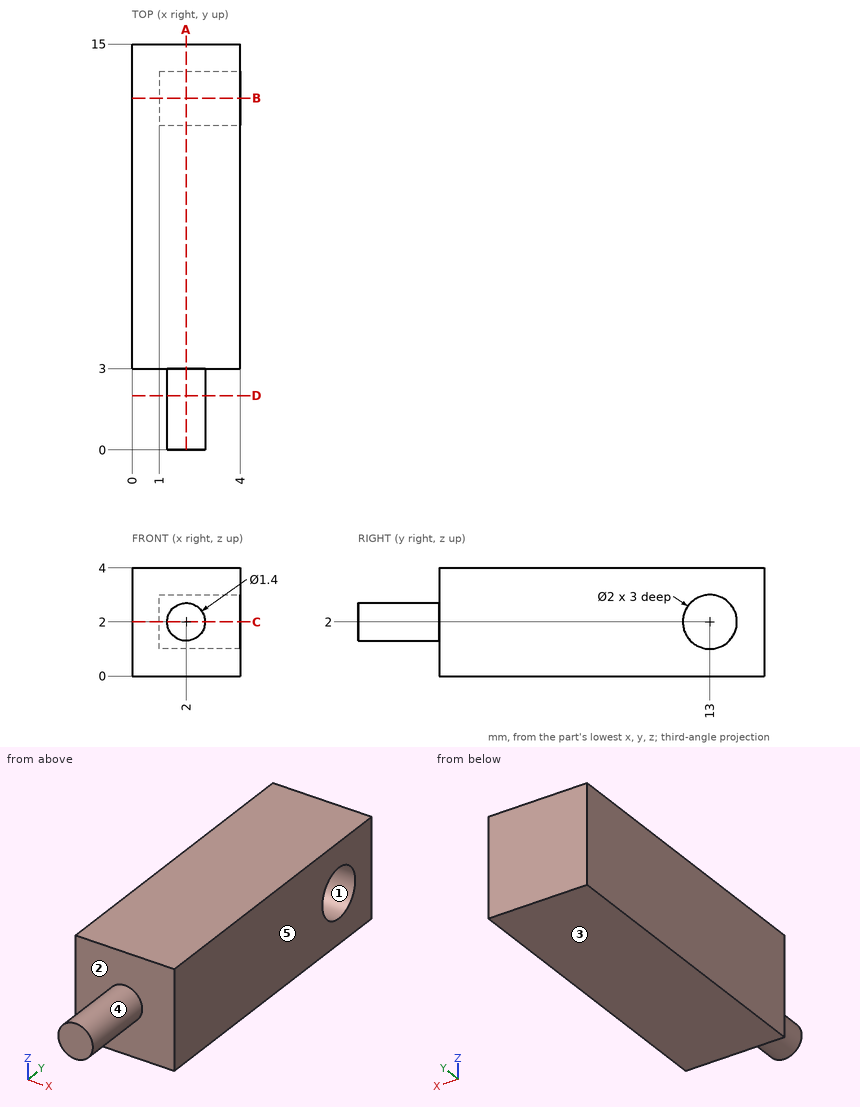
Geometry: see drawing. Coordinates: mm, zero at the bounding-box minimum. A direction names the side the tool comes from. Give positions to 0.01 mm unless a question says otherwise; leave off trailing zeros. Write each loop counter-clockwise with the first axis right and the second up, starting at its lowest first coordinate (ties: lowest second). Pieces come first, ordered by that corner, then holes. Notation, with made-up numbers: (-10.75, 8.25) - (-4.75, 8.25) arc R18 ccw to (-4.75, 42.25) - close; hole circle Ø11 at (34.25, 8.5). An arc over 180 degrees is marked (long way). Return JSON: item names as keys, results as strings. Group by question number.
1) Section C-C on z = 2. Return the cut outline in (x, y).
2) Section A-A on x = 2. Return the cut outline in (y, z).
3) Section D-D on y = 2. Return the cut outline in (x, z).
4) Set-up query: the marked faces 4 and 5. Return all of +Z, -Z, +X, -X, +Y, -Y with unobstructed straight access to the full face (end or side cutting, diameter ignored); none if empty.
5) First-contact query: P1, Ø1.6, axis at y = 13, z = 2, coming from the +X side. Flat tip, straight axial feed; report the tip coordinate or a pass-through.
6) Section B-B on y = 13. Return the cut outline in (x, z), plus the area to 4 significant figures.
7) Line query: line 1 (Y direction, x = 1.85, z = 2); line 2 (Y direction, x = 2.95, z = 2); line 3 (Z direction, x = 1.3, y = 13.5). Output: solid intervals per line, ascending.
8) Mould query, pull axis Z, two halves, no side actions, for the marked faces 1, 2 and 3. Classes: released by +Z, released by -Z, zero draft, split by the parting line, or undercut.
Filled in:
{
 "1": {"outline": "(0, 3) - (1.3, 3) - (1.3, 0) - (2.7, 0) - (2.7, 3) - (4, 3) - (4, 12) - (1, 12) - (1, 14) - (4, 14) - (4, 15) - (0, 15) - close"},
 "2": {"outline": "(0, 1.3) - (3, 1.3) - (3, 0) - (15, 0) - (15, 4) - (3, 4) - (3, 2.7) - (0, 2.7) - close; hole circle Ø2 at (13, 2)"},
 "3": {"outline": "circle Ø1.4 at (2, 2)"},
 "4": {"face 4": "-Y", "face 5": "+Z, -Z, +X, +Y, -Y"},
 "5": {"P1": "stops at x = 1"},
 "6": {"outline": "(0, 0) - (4, 0) - (4, 1) - (1, 1) - (1, 3) - (4, 3) - (4, 4) - (0, 4) - close", "area": "10.00 mm^2"},
 "7": {"line 1": "y = 0 to 12, 14 to 15", "line 2": "y = 3 to 12, 14 to 15", "line 3": "z = 0 to 1.13, 2.87 to 4"},
 "8": {"face 1": "undercut", "face 2": "zero draft", "face 3": "released by -Z"}
}
